Read the model definition and answer for the solid it produces. Units are mm, in the model's axes. A direction names the side the tool comes from. Coordinates: 2 decimals unless noted, no trailing zeros. Order: outer loops, then holes, each group sorted by start corner. A loop starts at its lowest first (then second) coordinate and runs counter-clockwise, first axis right, second up.
```python
from build123d import *

# Parameters (mm, degrees)
SKETCH1_W                = 7.25
SKETCH1_H                = 6.65
BASE_EXTRUDE_DEPTH       = 3.5052
CHAMFER1_SIZE            = 1.651
CHAMFER1_SIZE2           = 0.291115845
CHAMFER1_PART_2_SIZE     = 1.651
CHAMFER1_PART_2_SIZE2    = 0.291115845
CHAMFER1_PART_3_SIZE     = 1.651
CHAMFER1_PART_3_SIZE2    = 0.291115845
CHAMFER1_PART_4_SIZE     = 1.651
CHAMFER1_PART_4_SIZE2    = 0.291115845
CHAMFER2_SIZE            = 1.651
CHAMFER2_SIZE2           = 0.291115845
CHAMFER2_PART_2_SIZE     = 1.651
CHAMFER2_PART_2_SIZE2    = 0.291115845
CHAMFER2_PART_3_SIZE     = 1.651
CHAMFER2_PART_3_SIZE2    = 0.291115845
CHAMFER2_PART_4_SIZE     = 1.651
CHAMFER2_PART_4_SIZE2    = 0.291115845
SKETCH3_R                = 0.5
CUT_EXTRUDE1_DEPTH       = 0.3
BOSS_EXTRUDE_THIN3_DEPTH = 0.5969
LPATTERN1_COUNT          = 3
LPATTERN1_PITCH          = 2.54
MIRROR1_COPY_1_DEPTH     = 0.5969
MIRROR1_COPY_2_DEPTH     = 0.5969
FILLET_1_R               = 0.2


with BuildPart() as part:
    # Sketch1 → Base-Extrude (new body)
    with BuildSketch(Plane.XY):
        with Locations((2.99, 4.214)):
            Rectangle(SKETCH1_W, SKETCH1_H)
    extrude(amount=BASE_EXTRUDE_DEPTH)

    # Chamfer1
    chamfer1_edges = [part.edges().sort_by_distance(p)[0] for p in [
        (6.615, 4.214, 3.5052),
    ]]
    chamfer1_side = [part.faces().sort_by_distance(p)[0] for p in [
        (6.615, 4.214, 1.7526),
    ]]
    chamfer(chamfer1_edges, length=CHAMFER1_SIZE, length2=CHAMFER1_SIZE2, reference=chamfer1_side[0])

    # Chamfer1 part 2
    chamfer1_part_2_edges = [part.edges().sort_by_distance(p)[0] for p in [
        (2.99, 7.539, 3.5052),
    ]]
    chamfer1_part_2_side = [part.faces().sort_by_distance(p)[0] for p in [
        (2.99, 7.539, 1.7526),
    ]]
    chamfer(chamfer1_part_2_edges, length=CHAMFER1_PART_2_SIZE, length2=CHAMFER1_PART_2_SIZE2, reference=chamfer1_part_2_side[0])

    # Chamfer1 part 3
    chamfer1_part_3_edges = [part.edges().sort_by_distance(p)[0] for p in [
        (-0.635, 4.214, 3.5052),
    ]]
    chamfer1_part_3_side = [part.faces().sort_by_distance(p)[0] for p in [
        (-0.635, 4.214, 1.7526),
    ]]
    chamfer(chamfer1_part_3_edges, length=CHAMFER1_PART_3_SIZE, length2=CHAMFER1_PART_3_SIZE2, reference=chamfer1_part_3_side[0])

    # Chamfer1 part 4
    chamfer1_part_4_edges = [part.edges().sort_by_distance(p)[0] for p in [
        (2.99, 0.889, 3.5052),
    ]]
    chamfer1_part_4_side = [part.faces().sort_by_distance(p)[0] for p in [
        (2.99, 0.889, 1.7526),
    ]]
    chamfer(chamfer1_part_4_edges, length=CHAMFER1_PART_4_SIZE, length2=CHAMFER1_PART_4_SIZE2, reference=chamfer1_part_4_side[0])

    # Chamfer2
    chamfer2_edges = [part.edges().sort_by_distance(p)[0] for p in [
        (2.99, 7.539, 0),
    ]]
    chamfer2_side = [part.faces().sort_by_distance(p)[0] for p in [
        (2.99, 7.539, 0.9271),
    ]]
    chamfer(chamfer2_edges, length=CHAMFER2_SIZE, length2=CHAMFER2_SIZE2, reference=chamfer2_side[0])

    # Chamfer2 part 2
    chamfer2_part_2_edges = [part.edges().sort_by_distance(p)[0] for p in [
        (6.615, 4.214, 0),
    ]]
    chamfer2_part_2_side = [part.faces().sort_by_distance(p)[0] for p in [
        (6.615, 4.214, 0.9271),
    ]]
    chamfer(chamfer2_part_2_edges, length=CHAMFER2_PART_2_SIZE, length2=CHAMFER2_PART_2_SIZE2, reference=chamfer2_part_2_side[0])

    # Chamfer2 part 3
    chamfer2_part_3_edges = [part.edges().sort_by_distance(p)[0] for p in [
        (2.99, 0.889, 0),
    ]]
    chamfer2_part_3_side = [part.faces().sort_by_distance(p)[0] for p in [
        (2.99, 0.889, 0.9271),
    ]]
    chamfer(chamfer2_part_3_edges, length=CHAMFER2_PART_3_SIZE, length2=CHAMFER2_PART_3_SIZE2, reference=chamfer2_part_3_side[0])

    # Chamfer2 part 4
    chamfer2_part_4_edges = [part.edges().sort_by_distance(p)[0] for p in [
        (-0.635, 4.214, 0),
    ]]
    chamfer2_part_4_side = [part.faces().sort_by_distance(p)[0] for p in [
        (-0.635, 4.214, 0.9271),
    ]]
    chamfer(chamfer2_part_4_edges, length=CHAMFER2_PART_4_SIZE, length2=CHAMFER2_PART_4_SIZE2, reference=chamfer2_part_4_side[0])

    # Sketch3 → Cut-Extrude1 (cut)
    with BuildSketch(Plane(origin=(0.118935742, 0.142956615, 3.5052), x_dir=(1, 0, 0), z_dir=(0, 0, 1))):
        with Locations((0.349775267, 1.734053999)):
            Circle(SKETCH3_R)
    extrude(amount=-CUT_EXTRUDE1_DEPTH, mode=Mode.SUBTRACT)

    # Sketch4 → Boss-Extrude-Thin3 (add, symmetric)
    with BuildSketch(Plane.ZY.offset(-0.45)):
        with BuildLine():
            Line((1.651, 0.889), (1.651, 0.552741678))
            ThreePointArc((1.651, 0.552741678), (1.61148335, 0.433388864), (1.508549057, 0.361200283))
            Line((1.508549057, 0.361200283), (-0.057549057, -0.109337536))
            ThreePointArc((-0.057549057, -0.109337536), (-0.16048335, -0.181526117), (-0.2, -0.300878931))
            Line((-0.2, -0.300878931), (-0.2, -0.686))
            Line((-0.2, -0.686), (0.05, -0.686))
            Line((0.05, -0.686), (0.05, -0.33806435))
            Line((0.05, -0.33806435), (1.580485379, 0.121773539))
            ThreePointArc((1.580485379, 0.121773539), (1.812087538, 0.284197846), (1.901, 0.552741678))
            Line((1.901, 0.552741678), (1.901, 0.889))
            Line((1.901, 0.889), (1.651, 0.889))
        make_face()
    boss_extrude_thin3 = extrude(amount=BOSS_EXTRUDE_THIN3_DEPTH, both=True)

    # LPattern1: Boss-Extrude-Thin3 ×3
    with Locations(*[(i * LPATTERN1_PITCH, 0, 0) for i in range(1, LPATTERN1_COUNT)]):
        add(boss_extrude_thin3)

    # Mirror1: Boss-Extrude-Thin3 across plane
    add(boss_extrude_thin3.mirror(Plane(origin=(0, 4.214, 0), x_dir=(0, 0, 1), z_dir=(0, -1, 0))))

    # Mirror1 copy 1 sketch → Mirror1 copy 1 (add, symmetric)
    with BuildSketch(Plane(origin=(2.99, 8.428, 0), x_dir=(0, 0, 1), z_dir=(-1, 0, 0))):
        with BuildLine():
            Line((1.651, -0.889), (1.651, -0.552741678))
            ThreePointArc((1.651, -0.552741678), (1.61148335, -0.433388864), (1.508549057, -0.361200283))
            Line((1.508549057, -0.361200283), (-0.057549057, 0.109337536))
            ThreePointArc((-0.057549057, 0.109337536), (-0.16048335, 0.181526117), (-0.2, 0.300878931))
            Line((-0.2, 0.300878931), (-0.2, 0.686))
            Line((-0.2, 0.686), (0.05, 0.686))
            Line((0.05, 0.686), (0.05, 0.33806435))
            Line((0.05, 0.33806435), (1.580485379, -0.121773539))
            ThreePointArc((1.580485379, -0.121773539), (1.812087538, -0.284197846), (1.901, -0.552741678))
            Line((1.901, -0.552741678), (1.901, -0.889))
            Line((1.901, -0.889), (1.651, -0.889))
        make_face()
    extrude(amount=MIRROR1_COPY_1_DEPTH, both=True)

    # Mirror1 copy 2 sketch → Mirror1 copy 2 (add, symmetric)
    with BuildSketch(Plane(origin=(5.53, 8.428, 0), x_dir=(0, 0, 1), z_dir=(-1, 0, 0))):
        with BuildLine():
            Line((1.651, -0.889), (1.651, -0.552741678))
            ThreePointArc((1.651, -0.552741678), (1.61148335, -0.433388864), (1.508549057, -0.361200283))
            Line((1.508549057, -0.361200283), (-0.057549057, 0.109337536))
            ThreePointArc((-0.057549057, 0.109337536), (-0.16048335, 0.181526117), (-0.2, 0.300878931))
            Line((-0.2, 0.300878931), (-0.2, 0.686))
            Line((-0.2, 0.686), (0.05, 0.686))
            Line((0.05, 0.686), (0.05, 0.33806435))
            Line((0.05, 0.33806435), (1.580485379, -0.121773539))
            ThreePointArc((1.580485379, -0.121773539), (1.812087538, -0.284197846), (1.901, -0.552741678))
            Line((1.901, -0.552741678), (1.901, -0.889))
            Line((1.901, -0.889), (1.651, -0.889))
        make_face()
    extrude(amount=MIRROR1_COPY_2_DEPTH, both=True)

    # Скругление1
    fillet_1_edges = [part.edges().sort_by_distance(p)[0] for p in [
        (-0.343884155, 4.214, 3.5052),
        (2.99, 7.247884155, 3.5052),
        (6.323884155, 4.214, 3.5052),
        (2.99, 1.180115845, 3.5052),
        (-0.343884155, 4.214, 0),
        (2.99, 7.247884155, 0),
        (6.323884155, 4.214, 0),
        (2.99, 1.180115845, 0),
    ]]
    fillet(fillet_1_edges, radius=FILLET_1_R)


solid = part.part
```
1) A cutting plane is placed at B-B, the plane z = 0.95. Determine the outline of the cut face in (x, y).
A:
outline: (-0.51, 1.01) - (6.49, 1.01) - (6.49, 7.42) - (-0.51, 7.42) - close; (-0.15, -0.07) - (1.05, -0.07) - (1.05, 0.19) - (-0.15, 0.19) - close; (-0.15, 8.23) - (1.05, 8.23) - (1.05, 8.5) - (-0.15, 8.5) - close; (2.39, -0.07) - (3.59, -0.07) - (3.59, 0.19) - (2.39, 0.19) - close; (2.39, 8.23) - (3.59, 8.23) - (3.59, 8.5) - (2.39, 8.5) - close; (4.93, -0.07) - (6.13, -0.07) - (6.13, 0.19) - (4.93, 0.19) - close; (4.93, 8.23) - (6.13, 8.23) - (6.13, 8.5) - (4.93, 8.5) - close
2) A cutting plane is placed at A-A, the plane x = 4.25. Determine the outline of the cut face in (y, z), and give its area (3 significant figures).
A:
outline: (0.89, 1.65) - (1.15, 0.17) arc R0.2 ccw to (1.35, 0) - (7.08, 0) arc R0.2 ccw to (7.28, 0.17) - (7.54, 1.65) - (7.54, 1.85) - (7.28, 3.34) arc R0.2 ccw to (7.08, 3.51) - (1.35, 3.51) arc R0.2 ccw to (1.15, 3.34) - (0.89, 1.85) - close
area: 22.3 mm2
3) Determine the mould class of faces 1 (the flat face through (-0.5, 4.17, 2.61)), 2 (the flat face through (2.98, 0.13, 0.74)), 3 (the flat face through (5.522, -0.111, 0.805)) for opening direction Y: pulls with the +Y half, pulls with the -Y half, needs draft (parallel to the pull), parting line crosses it, or undercut.
A:
face 1: needs draft
face 2: undercut
face 3: pulls with the -Y half
4) Which of the six approach directions +Z, -Z, +X, -X, +Y, -Y give full straight-line access (tool end or side, diameter ignored) to faces 4 (the flat face through (0.5, 1.9, 3.205)), 5 (the flat face through (3, 4, 0))?
A:
face 4: +Z
face 5: -Z, +X, -X
5) Flat-ended cylindrical pins translate along their axes: pin 1 Ø1.7 at (y, z) = (0, 0.5) entering from -X; pin 2 Ø1.7 at (y, z) = (8.5, 1) entering from +X; pin 3 Ø1 at (x, y) = (1.5, 1) entering from -Z; pin 4 Ø2 at (y, z) = (6, 2.5) entering from +X (3 decimals). Find the tip coordinate at first contact, or state that the pin passes through.
A:
pin 1: stops at x = -0.15
pin 2: stops at x = 6.13
pin 3: stops at z = 0
pin 4: stops at x = 6.615
6) A cutting plane is placed at C-C, the plane y = 5. Determine the outline of the cut face in (x, z) (3 decimals).
A:
outline: (-0.635, 1.651) - (-0.373, 0.165) arc R0.2 ccw to (-0.176, 0) - (6.156, 0) arc R0.2 ccw to (6.353, 0.165) - (6.615, 1.651) - (6.615, 1.854) - (6.353, 3.34) arc R0.2 ccw to (6.156, 3.505) - (-0.176, 3.505) arc R0.2 ccw to (-0.373, 3.34) - (-0.635, 1.854) - close
7) Straight lines are drawn through the part: line 1 (Y direction, x = 3.5, z = 0.6); line 2 (X direction, y = 0.5, z = 1.7); line 3 (Y direction, x = 2.5, z = 1.4). For each, find the intervals that lie inside material, in ascending order.
A:
line 1: y = -0.17 to 0.09, 1.07 to 7.35, 8.34 to 8.6
line 2: x = -0.15 to 1.05, 2.39 to 3.59, 4.93 to 6.13
line 3: y = 0.07 to 0.33, 0.93 to 7.49, 8.1 to 8.36
